```python
from build123d import *

# Parameters (mm, degrees)
SKETCH_1_W               = 10
SKETCH_1_H               = 38
SKETCH_1_R               = 1.1
EXTRUDE_1_DEPTH          = 0.75
EXTRUDE_1_DEPTH_BACK     = 0.75
SKETCH_3_W               = 20
SKETCH_3_H               = 38.036879249
EXTRUDE_2_DEPTH          = 1.5
EXTRUDE_3_DEPTH          = 1
EXTRUDE_3_DEPTH_BACK     = 1
SKETCH_10_W              = 112.497058814
SKETCH_10_H              = 20.543414641
CUT_EXTRUDE_4_DEPTH      = 0.2
CUT_EXTRUDE_4_DEPTH_BACK = 0.2
SKETCH_11_W              = 104.514605189
SKETCH_11_H              = 21.657747512
CUT_EXTRUDE_5_DEPTH      = 0.2
CUT_EXTRUDE_5_DEPTH_BACK = 0.2
SKETCH_12_W              = 1.5
SKETCH_12_H              = 9
CUT_EXTRUDE_6_DEPTH      = 39


with BuildPart() as part:
    # Sketch 1 → Extrude 1 (new body, two sides)
    with BuildSketch(Plane.XY) as extrude_1_sk:
        with Locations((-4.101832994, 0.735234216)):
            Rectangle(SKETCH_1_W, SKETCH_1_H)
        with Locations((-6.601832994, -15.764765784)):
            Circle(SKETCH_1_R, mode=Mode.SUBTRACT)
        with Locations((-6.578411405, 17.235234216)):
            Circle(SKETCH_1_R, mode=Mode.SUBTRACT)
    extrude(amount=EXTRUDE_1_DEPTH)
    extrude(extrude_1_sk.sketch, amount=-EXTRUDE_1_DEPTH_BACK)

    # Sketch 3 → Extrude 2 (add)
    with BuildSketch(Plane(origin=(-0.5, 0, 0), x_dir=(0, 0, -1), z_dir=(1, 0, 0))):
        with Locations((0, 0.716794592)):
            Rectangle(SKETCH_3_W, SKETCH_3_H)
    extrude(amount=EXTRUDE_2_DEPTH)

    # Sketch 4 → Extrude 3 (add, two sides)
    with BuildSketch(Plane.XY) as extrude_3_sk:
        with BuildLine():
            Line((1, 19.735234216), (1, -18.298860138))
            ThreePointArc((1, -18.298860138), (51.989546932, -13.993809638), (101, 0.718187039))
            ThreePointArc((101, 0.718187039), (51.989546932, 15.430183716), (1, 19.735234216))
        make_face()
    extrude(amount=EXTRUDE_3_DEPTH)
    extrude(extrude_3_sk.sketch, amount=-EXTRUDE_3_DEPTH_BACK)

    # Sketch 10 → Cut-Extrude 4 (cut, two sides)
    with BuildSketch(Plane(origin=(0, 19.735234216, 0), x_dir=(1, 0, 0), z_dir=(0, 1, 0))) as cut_extrude_4_sk:
        with Locations((46.49437126, 0.271707321)):
            Rectangle(SKETCH_10_W, SKETCH_10_H)
    extrude(amount=CUT_EXTRUDE_4_DEPTH, mode=Mode.SUBTRACT)
    extrude(cut_extrude_4_sk.sketch, amount=-CUT_EXTRUDE_4_DEPTH_BACK, mode=Mode.SUBTRACT)

    # Sketch 11 → Cut-Extrude 5 (cut, two sides)
    with BuildSketch(Plane(origin=(0, -18.301645033, 0), x_dir=(-1, 0, 0), z_dir=(0, -1, 0))) as cut_extrude_5_sk:
        with Locations((-51.541283716, 0.828873756)):
            Rectangle(SKETCH_11_W, SKETCH_11_H)
    extrude(amount=CUT_EXTRUDE_5_DEPTH, mode=Mode.SUBTRACT)
    extrude(cut_extrude_5_sk.sketch, amount=-CUT_EXTRUDE_5_DEPTH_BACK, mode=Mode.SUBTRACT)

    # Sketch 12 → Cut-Extrude 6 (cut)
    with BuildSketch(Plane(origin=(0, 19.735234216, 0), x_dir=(1, 0, 0), z_dir=(0, 1, 0))):
        with Locations((0.25, -5.5)):
            Rectangle(SKETCH_12_W, SKETCH_12_H)
        with Locations((0.25, 5.5)):
            Rectangle(SKETCH_12_W, SKETCH_12_H)
    extrude(amount=-CUT_EXTRUDE_6_DEPTH, mode=Mode.SUBTRACT)


solid = part.part
```
For this review, take the finished solid that the model builds, in its own axes (mm). A direction names the side the tool comes from. Round coordinates to 2 decimals unless told otherwise and drop trailing zeros. Write each loop counter-clockwise with the first axis right and the second up, starting at its lowest first coordinate (ties: lowest second). Pieces come first, ordered by that corner, then holes.
1) Insertion check: pin 1 Ø3 at (x, y) = (-6.58, 17.24) entering from -Z; pin 2 Ø2.5 at (x, y) = (-6, 8.5) entering from +Z. Each pin has a flat end and moves straight along its axis. Give the tip position at first contact, or say it passes through.
Answer below:
pin 1: stops at z = -0.75
pin 2: stops at z = 0.75
2) For line 1 along Z through (x, y) = (-1, 4.5); line 2 along Y through (x, z) = (5.5, -0.3); line 3 along Y through (x, z) = (40, -0.75), list the stretches that pass through material, from the lowest coordinate up.
Answer below:
line 1: z = -0.75 to 0.75
line 2: y = -18.1 to 19.54
line 3: y = -15.97 to 17.41
3) Take a section at A-A on z = 0.15. Give the boundary of the cut face in (x, y).
Answer below:
outline: (-9.1, -18.26) - (-0.72, -18.26) - (-0.72, -18.1) - (16.79, -18.1) arc R247.18 ccw to (101, 0.72) arc R247.18 ccw to (16.85, 19.54) - (-9.1, 19.54) - close; hole circle Ø2.2 at (-6.6, -15.76); hole circle Ø2.2 at (-6.58, 17.24)
4) Take a section at B-B on y = -3. Give the boundary of the cut face in (x, z).
Answer below:
outline: (-9.1, -0.75) - (-0.5, -0.75) - (-0.5, -1) - (91.55, -1) - (91.55, 1) - (-0.5, 1) - (-0.5, 0.75) - (-9.1, 0.75) - close
5) Take a section at D-D on y = 3. Give the boundary of the cut face in (x, z), then the cut area to 3 significant figures.
Answer below:
outline: (-9.1, -0.75) - (-0.5, -0.75) - (-0.5, -1) - (95.34, -1) - (95.34, 1) - (-0.5, 1) - (-0.5, 0.75) - (-9.1, 0.75) - close
area: 205 mm2
6) Take a section at C-C on x = 49.5. Give the boundary of the cut face in (y, z), then the cut area to 3 significant figures.
Answer below:
outline: (-14.45, -1) - (15.89, -1) - (15.89, 1) - (-14.45, 1) - close
area: 60.7 mm2
7) Machinability: for faces 1 (the face through (-5, 1, -0.75)), 2 (the face through (-5, 1, 0.75)), 3 (the face through (59.131, -12.526, 0.014)), which of the approach directions +Z, -Z, +X, -X, +Y, -Y give a long, thin tool a straight path to every point of the face, cutting with its end or side? Answer none if there is none.
Answer below:
face 1: -Z, -X, +Y, -Y
face 2: +Z, -X, +Y, -Y
face 3: +Z, -Z, +X, -Y
8) Mouldability with a two-part tool opening along Y and no side actions: class faces 4 (the face through (-6.745, -14.674, -0.01)), 5 (the face through (-6.817, 16.161, -0.01)), 6 (the face through (38, 1, -1)), 7 (the face through (8, -18.102, 0)) as +Y half, -Y half, draft (parallel to the pull), parting line (faces both ways), or undercut.
Answer below:
face 4: undercut
face 5: undercut
face 6: draft
face 7: -Y half
